For this review, take the finished solid that the model builds, in its own axes (mm). Coordinates: 2 decimals unless noted, no trailing zeros. Loops run counter-clockwise (first coordinate to the right, second up) from the corner with the lowest first, then second, coordinate; pieces in that order, holes last. Notation, with made-up numbers: M -37,61.25 L -17,61.25 A10 ccw -17,73.25 Z; hole C 29,84 d5. An arc over 180 degrees is marked long. Put each result on its own line as item: value.
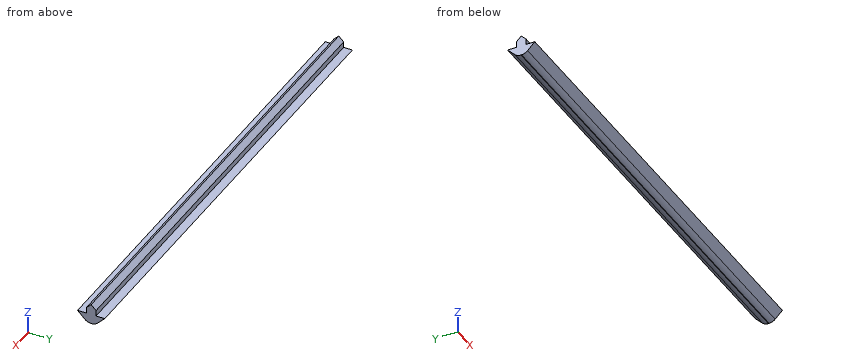
```python
from build123d import *

# Parameters (mm, degrees)
F0_W        = 76.2
F0_H        = 1.5875
F0_H_2      = 2.38125
F1_DEPTH    = 1.5875
F2_DEPTH    = 3.81
F3_T1_DEPTH = 82.7320747894
F4_T1_DEPTH = 89.2641495789
F5_R        = 1.397


# Not quite as in the source:
# - a fillet or chamfer that OpenCascade refuses, or shapes differently, is made with other operations: its cross-section is extruded or revolved along the edge and cut away or added


with BuildPart() as f1:
    # F0 (on Top) → F1 (new body)
    with BuildSketch(Plane.XY):
        Rectangle(F0_W, F0_H)
        with Locations((0, -1.984375)):
            Rectangle(F0_W, F0_H_2)
        with Locations((0, 1.984375)):
            Rectangle(F0_W, F0_H_2)
    extrude(amount=F1_DEPTH)

    # F0 (on Top) → F2 (join)
    with BuildSketch(Plane.XY):
        Rectangle(F0_W, F0_H)
    extrude(amount=F2_DEPTH)

    # F3: chamfer of 1.27 on 2 edges, made by hand

    # F3_s2 → F3_t1 (cut)
    with BuildSketch(Plane.YZ.offset(-41.3660373947)):
        Polygon((-0.79375, 2.54), (0.47625, 3.81), (-0.79375, 3.81), align=None)
        Polygon((-0.47625, 3.81), (0.79375, 2.54), (0.79375, 3.81), align=None)
    extrude(amount=F3_T1_DEPTH, mode=Mode.SUBTRACT)

    # F4: chamfer of 2.54 on 2 edges, made by hand

    # F4_s2 → F4_t1 (cut)
    with BuildSketch(Plane.YZ.offset(-44.6320747894)):
        Polygon((-3.175, 2.54), (-0.635, 0), (-3.175, 0), align=None)
        Polygon((0.635, 0), (3.175, 2.54), (3.175, 0), align=None)
    extrude(amount=F4_T1_DEPTH, mode=Mode.SUBTRACT)

    # F5
    f5_edges = [f1.edges().sort_by_distance(p)[0] for p in [
        (0, -0.635, 0),
        (0, 0.635, 0),
    ]]
    fillet(f5_edges, radius=F5_R)


solid = f1.part
```
(1) Wall thickness on line 1 along Y through (x, z) = (23, 2.15); line 2 along Z through (x, y) = (24.5, 1.95) (1 decimal); line 3 along Z through (x, y) = (28, -0.15): over which ranges is each line inside the solid? List them lowest first. Write a range as [from, to].
Determined:
line 1: y = [-0.79, 0.79]
line 2: z = [1.3, 1.6]
line 3: z = [0, 3.18]
(2) For pin 1 (1.5 mm diameter, centred on x = 20.5, z = 0.5, fed in from -Y) (3 decimals); pin 2 (1.1 mm diameter, centred on x = -5, y = -1.5, fed in from +Z); pin 3 (1.5 mm diameter, centred on x = -16.5, y = 1.5, fed in from +Z), all flat-tipped, find the tip position at first contact; note any pin that passes through.
Determined:
pin 1: stops at y = -1.885
pin 2: stops at z = 1.59
pin 3: stops at z = 2.58
(3) Add section A-A (x = -31). Write out the cut boundary in (y, z), plus the area to 3 significant figures.
Determined:
outline: M -2.22,1.59 L -1.04,0.41 A1.4 ccw -0.06,0 L 0.06,0 A1.4 ccw 1.04,0.41 L 2.22,1.59 L 0.79,1.59 L 0.79,2.54 L 0,3.33 L -0.79,2.54 L -0.79,1.59 Z
area: 6.59 mm^2
(4) Add section B-B (z = 1). Write out the cut boundary in (x, y) (3 decimals), plus the area to 3 significant figures.
Determined:
outline: M -38.1,-1.635 L 38.1,-1.635 L 38.1,1.635 L -38.1,1.635 Z
area: 249 mm^2
